Answer from the drawing. Dimensions are ordinates in mm from the lowest x, y and z of the part. A direction names the side the tool comes from. Coordinates: 2 decimals unless noted, no trailing zeros. Write each loop counter-clockwise with the first axis right and the second up, starting at its lowest first coordinate (ties: lowest second). Pieces come first, ordered by that corner, then holes. Notation, with made-up numbers: (53, 44) -> (58, 44) arc R13 cw to (58, 66) -> close; hole circle Ø6 at (-1.5, 0). An arc over 180 degrees is marked (long way). Use CSV: the item, a comma, the result in double quotes.
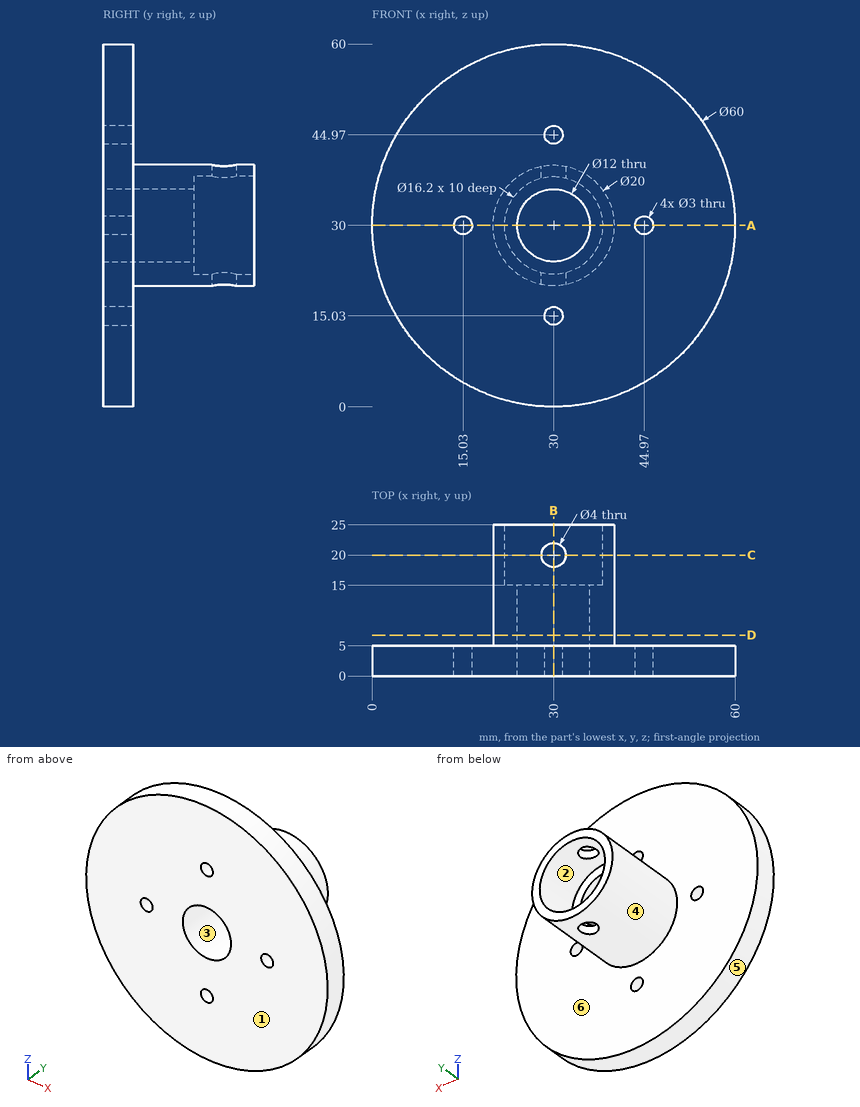
1. A cutting plane is placed at B-B (x = 30). Give the number of separate pieces and of enclosed holes in the cut face, and give its area (3 significant figures).
Solutions:
separate pieces,"6"
enclosed holes,"0"
area,"313 mm^2"
2. A cutting plane is placed at A-A (z = 30). Give the vertices of the cut face in (x, y), and give its area (3 significant figures).
Solutions:
outline,"(0, 0) -> (13.53, 0) -> (13.53, 5) -> (0, 5) -> close; (16.53, 0) -> (24, 0) -> (24, 15) -> (21.9, 15) -> (21.9, 25) -> (20, 25) -> (20, 5) -> (16.53, 5) -> close; (36, 0) -> (43.47, 0) -> (43.47, 5) -> (40, 5) -> (40, 25) -> (38.1, 25) -> (38.1, 15) -> (36, 15) -> close; (46.47, 0) -> (60, 0) -> (60, 5) -> (46.47, 5) -> close"
area,"328 mm^2"
3. Each of these flat-tipped pins is pushed along its axis until it touches: pin 1 Ø12 at (x, y) = (33.5, 14) entering from -Z; pin 2 Ø21 at (x, z) = (30, 30) entering from -Y; pin 3 Ø2.5 at (x, z) = (30, 44.97) entering from -Y; pin 4 Ø10 at (x, z) = (13, 38.5) entering from +Y. Where does it stop, or does it pass through?
Solutions:
pin 1,"stops at z = 20"
pin 2,"stops at y = 0"
pin 3,"passes through"
pin 4,"stops at y = 5"
4. A cutting plane is placed at D-D (y = 6.75). Give the vertices of the cut face in (x, z), and give its area (3 significant figures).
Solutions:
outline,"circle Ø20 at (30, 30); hole circle Ø12 at (30, 30)"
area,"201 mm^2"
5. A tool of negligible diameter and unlimited length cuts with its end or side. For the marked faces 5 and 6, from which of +Z, -Z, +X, -X, +Y, -Y can it reach the whole face along a straight path? Write none if from no direction.
Solutions:
face 5,"+Y, -Y"
face 6,"+Y"
6. Find the intervals of material crossed by line 1 along X through (y, z) = (2.4, 30); line 2 along X through (y, z) = (8.5, 30); line 3 along X through (y, z) = (21.75, 30), in increasing order.
Solutions:
line 1,"x = 0 to 13.53, 16.53 to 24, 36 to 43.47, 46.47 to 60"
line 2,"x = 20 to 24, 36 to 40"
line 3,"x = 20 to 21.9, 38.1 to 40"
7. For a pull along X with two mould halves and no side action, classify the marked faces 1, 2, 3 and 4 as pulls with the +X half, pulls with the -X half, needs draft (parallel to the pull), parting line crosses it, or undercut.
Solutions:
face 1,"needs draft"
face 2,"undercut"
face 3,"undercut"
face 4,"parting line crosses it"
8. A cutting plane is placed at C-C (y = 20). Give the vertices of the cut face in (x, z), and give its area (3 significant figures).
Solutions:
outline,"(28, 20.2) -> (28, 22.15) arc R8.1 cw to (28, 37.85) -> (28, 39.8) arc R10 ccw to start; (32, 20.2) arc R10 ccw to (32, 39.8) -> (32, 37.85) arc R8.1 cw to (32, 22.15) -> close"
area,"92.7 mm^2"
